Could you check a few things on this drawing? It's one solid part, dimensions in mm from its lowest x, y, z. A direction names the side the tool comes from. Round coordinates to 2 decimals unless told otherwise and drop trailing zeros. Order: outer loops, then holes, each group sorted by start corner. A loop starts at its lowest first (then second) coordinate and runs counter-clockwise, first axis right, second up. Notation, with made-up numbers: M -4,-21 L 44,-21 A22 ccw 44,-5 Z; hole C -12,-24 d6. An arc over 180 degrees is marked long. Answer as CSV lines item,"result". Start each with the question number.
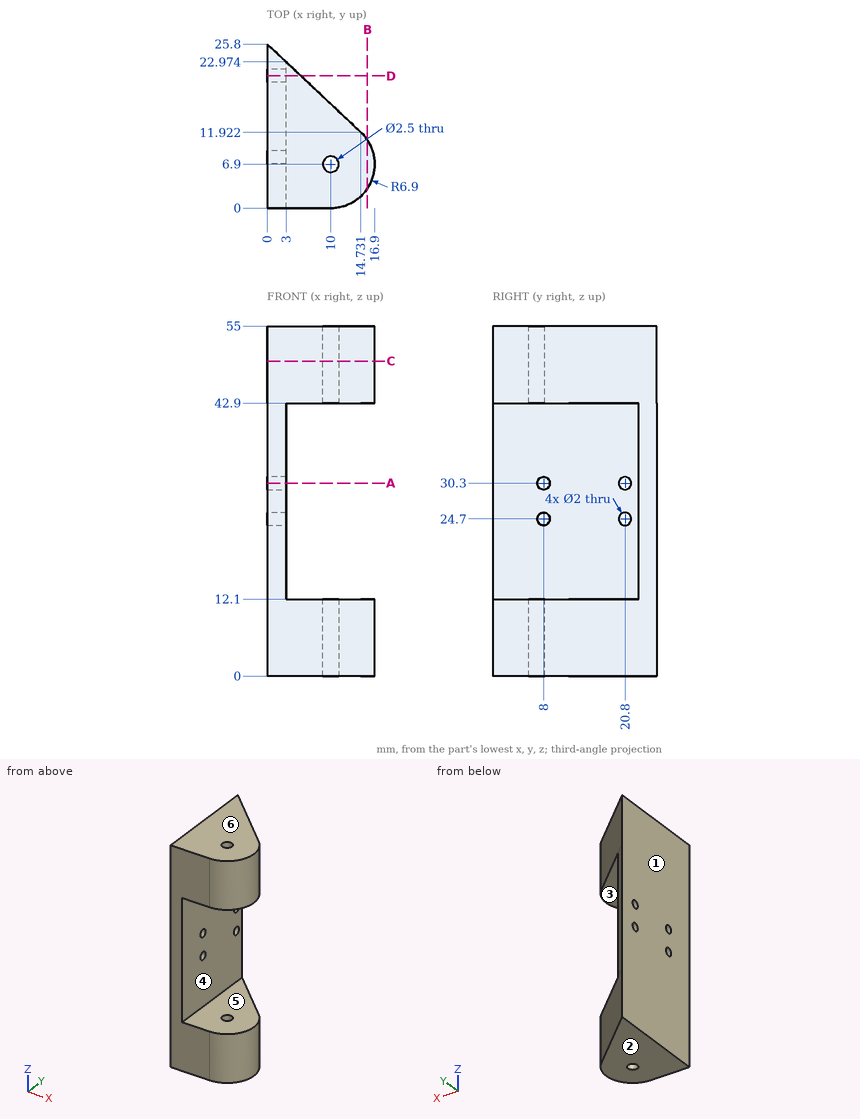
Item 1: If we section it at C-C on z = 49.5: Please give me the cut outline in (x, y).
Item 2: If we section it at B-B on x = 15.75: Please give me the cut outline in (y, z), and give its area (3 significant figures).
Item 3: For P1, Ø3, axis at y = 8, z = 30.3, coming from the +X side, with a flat end and sliding along its axis, tell me the tip position at first contact or that it passes through.
Item 4: If I drill on line 1 along Z through (x, y) = (2.3, 8); line 2 along Y through (x, z) = (1.75, 24.7); line 3 along Z through (x, y) = (16, 8.5), over which ranges is the centre line in solid material (lowest first)?
Item 5: Which directions (+Z, -Z, +X, -X, +Y, -Y) give clear straight access to the entire face, cutting with the end or side of a thin tool? Please do the marked faces 5 and 6.
Item 6: If we section it at D-D on y = 20.8: Please give me the cut outline in (x, z), and give its area (3 significant figures).
Item 7: We'd pull the mould along Z, two halves only. Please class the marked faces 1, 2, 3 and 4: pulls with the +Z half, pulls with the -Z half, needs draft (parallel to the pull), parting line crosses it, or undercut.
Item 8: If we section it at A-A on z = 30.3: Please give me the cut outline in (x, y).
Geometry says:
1,outline,"M 0,0 L 10,0 A6.9 ccw 14.73,11.92 L 0,25.8 Z; hole C 10,6.9 d2.5"
2,outline,"M 3.09,0 L 10.71,0 L 10.71,12.1 L 3.09,12.1 Z; M 3.09,42.9 L 10.71,42.9 L 10.71,55 L 3.09,55 Z"
2,area,"185 mm²"
3,P1,"x = 3"
4,line 1,"0 to 23.7, 25.7 to 29.3, 31.3 to 55"
4,line 2,"0 to 7, 9 to 19.8, 21.8 to 24.15"
4,line 3,"0 to 12.1, 42.9 to 55"
5,face 5,"+X, +Y, -Y"
5,face 6,"+Z, +X, -X, +Y, -Y"
6,outline,"M 0,0 L 5.31,0 L 5.31,12.1 L 3,12.1 L 3,23.7 L 0,23.7 Z; M 0,25.7 L 3,25.7 L 3,29.3 L 0,29.3 Z; M 0,31.3 L 3,31.3 L 3,42.9 L 5.31,42.9 L 5.31,55 L 0,55 Z"
6,area,"209 mm²"
7,face 1,"needs draft"
7,face 2,"pulls with the -Z half"
7,face 3,"undercut"
7,face 4,"undercut"
8,outline,"M 0,0 L 3,0 L 3,7 L 0,7 Z; M 0,9 L 3,9 L 3,19.8 L 0,19.8 Z; M 0,21.8 L 3,21.8 L 3,22.97 L 0,25.8 Z"
